Part model, mm, in its own coordinate system. A direction names the side the tool comes from. Coordinates: 2 decimals unless noted, no trailing zeros. Write each loop counter-clockwise with the first axis right and the second up, starting at its lowest first coordinate (ties: lowest second). Pieces come first, ordered by that corner, then holes. Notation, with made-up numbers: (30.5, -35) -> (36.5, -35) arc R22 ccw to (36.5, -27) -> close; hole circle Ø2 at (19, 9). An arc over 180 degrees is marked (long way). One line per question, with ' | ' between items. Start each with the question number.
Item 1: 3-axis set-ups, long thin cutter, end or side, ignore diameter. For faces 1 (the flat face through (-1, 1, 0)), 2 (the flat face through (-1, -26, -50.8)): which of +Z, -Z, +X, -X, +Y, -Y reach the whole face in a straight line?
Item 2: Saw through at A-A (y = 0). List the corners of the cut face in (x, z), and give its area (3 significant figures).
Item 3: Probe probe 1 along Z at (x, y) = (33.5, -20); probe 2 along Z at (x, y) = (3.5, 21); probe 3 along X at (y, z) = (17, -109.5). List the from-to ranges inside material, lowest first. Write a range as [from, to].
Item 4: Pin check, flat tips, straight feed: pin 1 (1 mm diameter, centred on x = -17.5, y = 30, fed in from -Z); pin 2 (12 mm diameter, centred on x = -9, y = -1.5, fed in from +Z); pin 3 (4 mm diameter, centred on x = -11, z = -75.5, fed in from -Y); pin 4 (1.5 mm diameter, centred on x = -19, z = -167.5, fed in from -Y). Stop position of each tip, or through.
Item 5: Saw through at C-C (z = -464). List the corners of the cut face in (x, y), and give its area (3 significant figures).
from build123d import *

# Parameters (mm, degrees)
F0_R     = 25.4
F1_DEPTH = 508
F0_R_2   = 44.45
F2_DEPTH = 50.8
F3_R     = 5.08


with BuildPart() as f1:
    # F0 (on Top) → F1 (new body)
    with BuildSketch(Plane.XY):
        Circle(F0_R)
    extrude(amount=-F1_DEPTH)

    # F0 (on Top) → F2 (join)
    with BuildSketch(Plane.XY):
        Circle(F0_R_2)
        Circle(F0_R, mode=Mode.SUBTRACT)
    extrude(amount=-F2_DEPTH)

    # F3
    f3_edges = [f1.edges().sort_by_distance(p)[0] for p in [
        (-44.45, 0, -50.8),
        (-44.45, 0, 0),
        (-25.4, 0, -508),
    ]]
    fillet(f3_edges, radius=F3_R)


solid = f1.part
From the geometry:
1) face 1: +Z, +X, -X, +Y, -Y | face 2: -Z
2) outline: (-44.45, -45.72) arc R5.08 ccw to (-39.37, -50.8) -> (-25.4, -50.8) -> (-25.4, -502.92) arc R5.08 ccw to (-20.32, -508) -> (20.32, -508) arc R5.08 ccw to (25.4, -502.92) -> (25.4, -50.8) -> (39.37, -50.8) arc R5.08 ccw to (44.45, -45.72) -> (44.45, -5.08) arc R5.08 ccw to (39.37, 0) -> (-39.37, 0) arc R5.08 ccw to (-44.45, -5.08) -> close | area: 27,700 mm2
3) probe 1: [-50.8, 0] | probe 2: [-507.91, 0] | probe 3: [-18.87, 18.87]
4) pin 1: z = -50.8 | pin 2: z = 0 | pin 3: y = -23.75 | pin 4: y = -17.67
5) outline: circle Ø50.8 at (0, 0) | area: 2,030 mm2
